For this review, use the dimensioned drawing (mm, ordinates from the lowest corner) and the shaded views. A direction names the side the tool comes from. Round coordinates to 2 decimals unless told otherwise and drop trailing zeros. Order: outer loops, then holes, each group sorted by start corner. A loop starts at its lowest first (then second) coordinate and runs counter-clockwise, first axis right, second up. Notation, with made-up numbers: (61.5, 70) - (100.5, 70) arc R22 ccw to (100.5, 102) - close; hole circle Ø3 at (74, -5). An arc over 180 degrees is marked (long way). Write item = value, one per line.
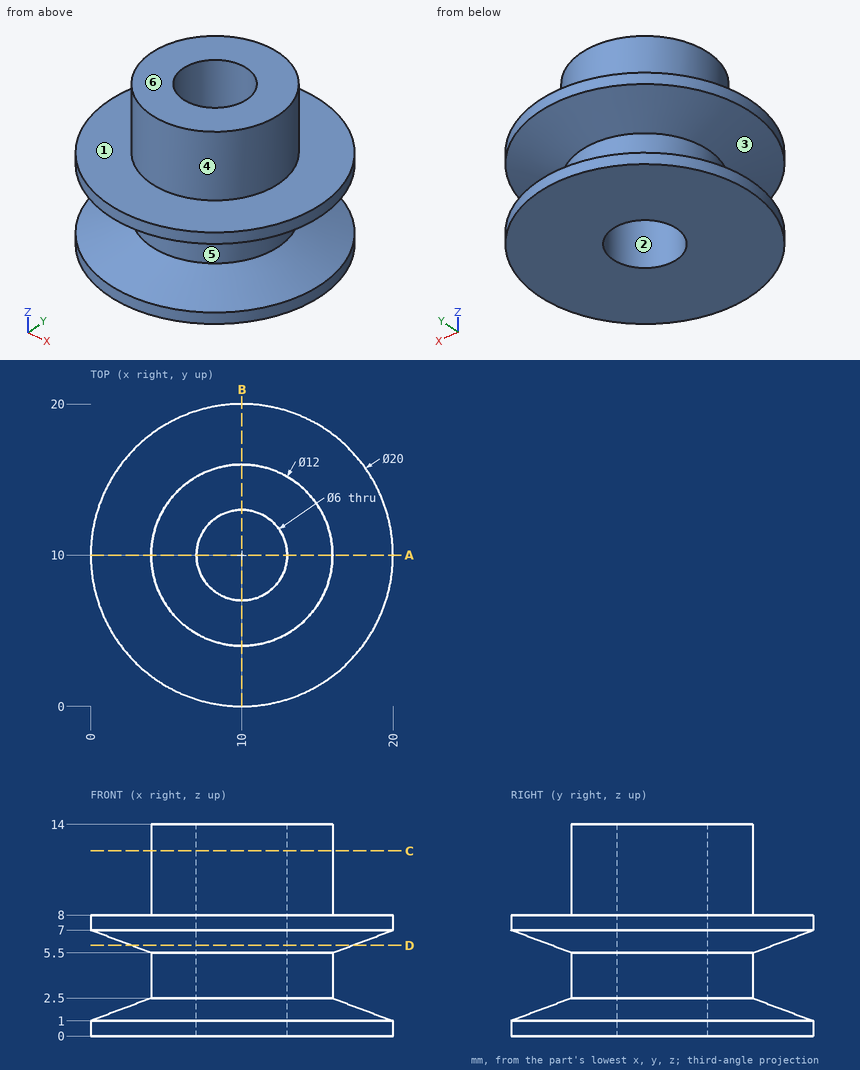
Item 1: Take a section at D-D, the plane z = 6. State the section outline as (x, y) points, and give its area (3 significant figures).
Data:
outline = circle Ø14.67 at (10, 10); hole circle Ø6 at (10, 10)
area = 141 mm2
Item 2: Insertion check: P1, Ø4, axis at x = 12.5, y = 3, coming from the +Z side; P2, Ø8, axis at y = 2.5, z = 9, coming from the -X side. Each pin has a flat end and moves straight along its axis. Give the tip position at first contact, or say it passes through.
Data:
P1 = 14
P2 = 0.68
Item 3: Take a section at A-A, the plane y = 10. State the section outline as (x, z) points, and give its area (3 significant figures).
Data:
outline = (0, 0) - (7, 0) - (7, 14) - (4, 14) - (4, 8) - (0, 8) - (0, 7) - (4, 5.5) - (4, 2.5) - (0, 1) - close; (13, 0) - (20, 0) - (20, 1) - (16, 2.5) - (16, 5.5) - (20, 7) - (20, 8) - (16, 8) - (16, 14) - (13, 14) - close
area = 112 mm2
Item 4: The part is to be moulded in two halves that separate along Z. For the marked faces 1, 2 and 3, say which applies: +Z half, -Z half, draft (parallel to the pull), parting line (faces both ways), or undercut.
Data:
face_1 = +Z half
face_2 = draft
face_3 = undercut
Item 5: Take a section at C-C, the plane z = 12.25. State the section outline as (x, y) points, and give its area (3 significant figures).
Data:
outline = circle Ø12 at (10, 10); hole circle Ø6 at (10, 10)
area = 84.8 mm2
Item 6: For the marked faces 4, 5 and 6, list the 3-axis set-ups (+Z, -Z, +X, -X, +Y, -Y) from which the entire face can be reached by the end or side of a thin tool; tool diameter is ignored.
Data:
face_4 = +Z
face_5 = none
face_6 = +Z, +X, -X, +Y, -Y
Item 7: For line 1 along X through (y, z) = (10, 8.25); line 2 along Y through (x, z) = (7.5, 9), list the stretches that pass through material, from the lowest coordinate up. Write a range as [from, to].
Data:
line_1 = [4, 7], [13, 16]
line_2 = [4.55, 8.34], [11.66, 15.45]
